Autodesk Inventor part; units mm, degrees
ref_plane "YZ Plane" through (0, 0, 0) normal (1, 0, 0) x (0, 1, 0)
ref_plane "XZ Plane" through (0, 0, 0) normal (0, 1, 0) x (-1, 0, 0)
ref_plane "XY Plane" through (0, 0, 0) normal (0, 0, 1) x (1, 0, 0)
sketch "Sketch1" plane through (0, 0, 0) normal (0, 0, 1) x (1, 0, 0)
  line L0 (0, 0) -> (127, 0)
  line L1 (127, 0) -> (127, 127)
  line L2 (127, 127) -> (0, 127)
  line L3 (0, 127) -> (0, 0)
  circle A0 centre (63.5, 63.5) radius 14.2875
  dimension "d0" = 127
  dimension "d1" = 127
  dimension "d2" = 28.575
extrude "Extrusion1" add sketch "Sketch1" along normal blind 3.175
sketch "Sketch2" plane through (0, 0, 3.175) normal (0, 0, 1) x (1, 0, 0)
  circle A0 centre (63.5, 114.3) radius 3.175
  line L0 (0, 127) -> (0, 0)
  line L1 (127, 127) -> (0, 127)
  dimension "d5" = 6.35
  dimension "d6" = 63.5
  dimension "d7" = 12.7
extrude "Extrusion2" cut sketch "Sketch2" against normal blind 3.175
properties part number "TestPlate"
For this review, take the finished solid that the model builds, in its own axes (mm). Round coordinates to 2 decimals unless told otherwise and drop trailing zeros. Order: outer loops, then holes, each group sorted by start corner. A loop starts at its lowest first (then second) coordinate and runs counter-clockwise, first axis right, second up. Notation, with made-up numbers: (23.5, 19) -> (74.5, 19) arc R21 ccw to (74.5, 48) -> close; hole circle Ø3 at (41.5, 0). An arc over 180 degrees is marked (long way). Use a Markdown table: item, result.
Item 1: For line 1 along Y through (x, z) = (63.5, 2.1) (1 decimal); line 2 along X through (y, z) = (66.5, 0.4), list the stretches that pass through material, from the lowest coordinate up. Write a range as [from, to].
Resolved:
| item | result |
|---|---|
| line 1 | y = [0, 49.2], [77.8, 111.1], [117.5, 127] |
| line 2 | x = [0, 49.53], [77.47, 127] |
Item 2: Take a section at D-D (y = 63.5). State the section outline as (x, z) points (1 decimal), plus the area to 4 significant figures.
Resolved:
| item | result |
|---|---|
| outline | (0, 0) -> (49.2, 0) -> (49.2, 3.2) -> (0, 3.2) -> close; (77.8, 0) -> (127, 0) -> (127, 3.2) -> (77.8, 3.2) -> close |
| area | 312.5 mm² |
Item 3: For pin 1 (5 mm diameter, centred on x = 63.5, y = 114.3, fed in from -Z); pin 2 (4 mm diameter, centred on x = 25.5, y = 24, fed in from -Z), all flat-tipped, find the tip position at first contact; note any pin that passes through.
Resolved:
| item | result |
|---|---|
| pin 1 | passes through |
| pin 2 | stops at z = 0 |
Item 4: Take a section at B-B (x = 63.5). State the section outline as (y, z) points (1 decimal).
Resolved:
| item | result |
|---|---|
| outline | (0, 0) -> (49.2, 0) -> (49.2, 3.2) -> (0, 3.2) -> close; (77.8, 0) -> (111.1, 0) -> (111.1, 3.2) -> (77.8, 3.2) -> close; (117.5, 0) -> (127, 0) -> (127, 3.2) -> (117.5, 3.2) -> close |
Item 5: Take a section at A-A (y = 114.3). State the section outline as (x, z) points (3 decimals).
Resolved:
| item | result |
|---|---|
| outline | (0, 0) -> (60.325, 0) -> (60.325, 3.175) -> (0, 3.175) -> close; (66.675, 0) -> (127, 0) -> (127, 3.175) -> (66.675, 3.175) -> close |
Item 6: Draft analysis for pull direction X (two halves, no side actions). For faces 1 (the cylindrical face through (65, 111.5, 1.6)), 2 (the flat face through (64, 127, 2)), 3 (the cylindrical face through (61.64, 49.334, 1.565)), 4 (the flat face through (0, 64, 2)), state which applies: +X half, -X half, draft (parallel to the pull), parting line (faces both ways), or undercut.
Resolved:
| item | result |
|---|---|
| face 1 | undercut |
| face 2 | draft |
| face 3 | undercut |
| face 4 | -X half |
Item 7: Take a section at C-C (z = 0.95). State how many separate pieces and enclosed holes the cut face has, plus the area to 3 significant figures.
Resolved:
| item | result |
|---|---|
| separate pieces | 1 |
| enclosed holes | 2 |
| area | 15,500 mm² |
